```python
from build123d import *

# Parameters (mm, degrees)
SKETCH1_W               = 34.925
SKETCH1_H               = 25.4
BOSS_EXTRUDE1_DEPTH     = 2.54
CUT_EXTRUDE3_DEPTH      = 44.259302179
CUT_EXTRUDE3_DEPTH_BACK = 44.259302179
SKETCH2_R               = 1.74625
SKETCH5_R               = 1.1303
CUT_EXTRUDE4_DEPTH      = 44.259302179
SKETCH6_W               = 10.16
SKETCH6_H               = 8.89
BOSS_EXTRUDE2_DEPTH     = 2.54
SKETCH7_W               = 6.985
SKETCH7_H               = 1.6002
CUT_EXTRUDE5_DEPTH      = 51.385559439
FILLET1_R               = 2.54
FILLET2_R               = 1.5875
FILLET3_R               = 2.54


with BuildPart() as part:
    # Sketch1 → Boss-Extrude1 (new body)
    with BuildSketch(Plane(origin=(0, 0, 0), x_dir=(1, 0, 0), z_dir=(0, 1, 0))):
        with Locations((17.4625, 12.7)):
            Rectangle(SKETCH1_W, SKETCH1_H)
    extrude(amount=BOSS_EXTRUDE1_DEPTH)

    # Sketch2 → Cut-Extrude3 (cut, two sides: drawn at the far end of the back side and taken through both)
    with BuildSketch(Plane(origin=(0, 2.54, 0), x_dir=(1, 0, 0), z_dir=(0, 1, 0)).offset(-CUT_EXTRUDE3_DEPTH_BACK)):
        with Locations(Location((3.81, 18.415, 0), (0, 0, 90))):
            Circle(SKETCH2_R)
        with Locations(Location((3.81, 6.985, 0), (0, 0, 90))):
            Circle(SKETCH2_R)
    extrude(amount=CUT_EXTRUDE3_DEPTH + CUT_EXTRUDE3_DEPTH_BACK, mode=Mode.SUBTRACT)

    # Sketch5 → Cut-Extrude4 (cut, through all)
    with BuildSketch(Plane(origin=(0, 2.54, 0), x_dir=(1, 0, 0), z_dir=(0, 1, 0))):
        with Locations(Location((31.75, 20.32, 0), (0, 0, 270))):
            Circle(SKETCH5_R)
        with Locations(Location((31.75, 5.08, 0), (0, 0, 90))):
            Circle(SKETCH5_R)
    extrude(amount=-CUT_EXTRUDE4_DEPTH, mode=Mode.SUBTRACT)

    # Sketch6 → Boss-Extrude2 (add)
    with BuildSketch(Plane(origin=(0, 2.54, 0), x_dir=(1, 0, 0), z_dir=(0, 1, 0))):
        with Locations((31.75, 29.845)):
            Rectangle(SKETCH6_W, SKETCH6_H)
    extrude(amount=-BOSS_EXTRUDE2_DEPTH)

    # Sketch7 → Cut-Extrude5 (cut, through all)
    with BuildSketch(Plane(origin=(0, 2.54, 0), x_dir=(1, 0, 0), z_dir=(0, 1, 0))):
        with Locations((31.75, 31.913620935)):
            Rectangle(SKETCH7_W, SKETCH7_H)
    extrude(amount=-CUT_EXTRUDE5_DEPTH, mode=Mode.SUBTRACT)

    # Fillet1
    # the kernel refuses this fillet: 2.54 mm, written as the material it adds along each edge
    with BuildSketch(Plane(origin=(26.67, 2.54, -25.4), x_dir=(-1, 0, 0), z_dir=(0, -1, 0))) as fillet1_piece_1:
        with BuildLine():
            CenterArc((FILLET1_R, FILLET1_R), FILLET1_R, 180, 90)
            Line((0, FILLET1_R), (-FILLET1_R * 0.02, FILLET1_R))
            Line((-FILLET1_R * 0.02, FILLET1_R), (-FILLET1_R * 0.02, -FILLET1_R * 0.02))
            Line((-FILLET1_R * 0.02, -FILLET1_R * 0.02), (FILLET1_R, -FILLET1_R * 0.02))
            Line((FILLET1_R, -FILLET1_R * 0.02), (FILLET1_R, 0))
        make_face()
    extrude(amount=2.54)
    with BuildSketch(Plane(origin=(34.925, 0, -25.4), x_dir=(0, 0, 1), z_dir=(0, 1, 0))) as fillet1_piece_2:
        with BuildLine():
            CenterArc((2.459344425, 2.54), FILLET1_R, 194.477512186, 75.522487814)
            Line((0, 1.905), (-0.049186888, 1.8923))
            ThreePointArc((-0.049186888, 1.8923), (-0.0508, 0.9525), (-0.0508, 0))
            Line((-0.0508, 0), (0, -0.0508))
            Line((0, -0.0508), (2.459344425, -0.0508))
            Line((2.459344425, -0.0508), (2.459344425, 0))
        make_face()
    extrude(amount=2.54)

    # Fillet2
    fillet2_edges = [part.edges().sort_by_distance(p)[0] for p in [
        (26.67, 1.27, -34.29),
        (36.83, 1.27, -34.29),
        (36.83, 1.27, -25.4),
    ]]
    fillet(fillet2_edges, radius=FILLET2_R)

    # Fillet3
    fillet3_edges = [part.edges().sort_by_distance(p)[0] for p in [
        (0, 1.27, -25.4),
        (34.925, 1.27, 0),
        (0, 1.27, 0),
    ]]
    fillet(fillet3_edges, radius=FILLET3_R)


solid = part.part
```
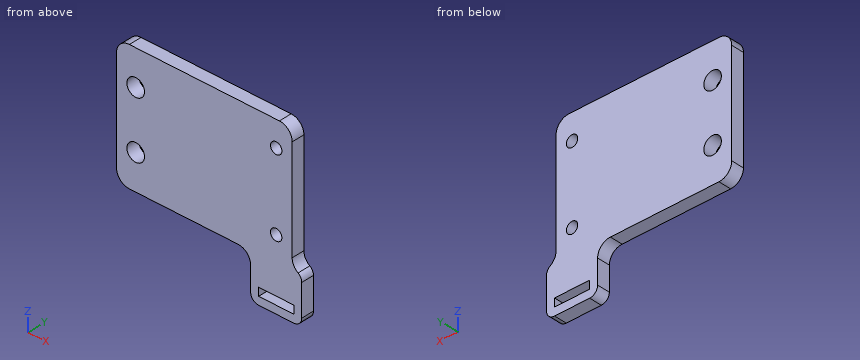
The model under review builds one solid part; all positions refer to its coordinate system, in mm. Round coordinates to 2 decimals unless told otherwise and drop trailing zeros. Write each loop counter-clockwise with the first axis right and the second up, starting at its lowest first coordinate (ties: lowest second). Pieces come first, ordered by that corner, then holes. Notation, with made-up numbers: (24.25, 5) -> (66.25, 5) arc R18 cw to (66.25, 21) -> close; hole circle Ø11 at (-26, -14.5). An arc over 180 degrees is marked (long way). Use CSV: the item, a comma, the result in double quotes.
Q1. To check wall thickness, follow probe 1 along X at (y, z) = (1.25, -32); probe 2 along Z at (x, y) = (3, 1.7); probe 3 along X at (y, z) = (1.9, -20.32) (3 decimals). State the ranges of each line that lie inside material, in increasing order. Write a range as [from, to].
Checks:
probe 1,"[26.67, 28.26], [35.24, 36.83]"
probe 2,"[-25.4, -19.96], [-16.87, -8.53], [-5.44, 0]"
probe 3,"[0, 30.62], [32.88, 34.925]"
Q2. Consider section B-B (x = 31.75). Give the boundary of the cut face in (y, z).
Checks:
outline,"(0, -34.29) -> (2.54, -34.29) -> (2.54, -32.71) -> (0, -32.71) -> close; (0, -31.11) -> (2.54, -31.11) -> (2.54, -21.45) -> (0, -21.45) -> close; (0, -19.19) -> (2.54, -19.19) -> (2.54, -6.21) -> (0, -6.21) -> close; (0, -3.95) -> (2.54, -3.95) -> (2.54, 0) -> (0, 0) -> close"
Q3. Consider section C-C (z = -32). Give the boundary of the cut face in (x, y).
Checks:
outline,"(26.67, 0) -> (28.26, 0) -> (28.26, 2.54) -> (26.67, 2.54) -> close; (35.24, 0) -> (36.83, 0) -> (36.83, 2.54) -> (35.24, 2.54) -> close"
Q4. For pin 1 Ø0.5 at (y, z) = (1.5, -32) entering from -X; pin 2 Ø1 at (y, z) = (1.5, -13) entering from +X (3 decimals), all flat-tipped, find the tip position at first contact; note any pin that passes through.
Checks:
pin 1,"x = 26.67"
pin 2,"x = 34.925"
Q5. Consider section D-D (y = 0.5). State how many separate pieces and enclosed holes the cut face has, then the cut area to 3 significant figures.
Checks:
separate pieces,"1"
enclosed holes,"5"
area,"936 mm²"
Q6. Consider section A-A (x = 3.81). Give the boundary of the cut face in (y, z), then the cut area to 3 significant figures.
Checks:
outline,"(0, -25.4) -> (2.54, -25.4) -> (2.54, -20.16) -> (0, -20.16) -> close; (0, -16.67) -> (2.54, -16.67) -> (2.54, -8.73) -> (0, -8.73) -> close; (0, -5.24) -> (2.54, -5.24) -> (2.54, 0) -> (0, 0) -> close"
area,"46.8 mm²"
